Here's how the part is built. I have some questions about the finished solid (model axes, mm). A direction names the side the tool comes from. Round coordinates to 2 decimals unless told otherwise and drop trailing zeros. Write each loop counter-clockwise with the first axis right and the second up, starting at its lowest first coordinate (ties: lowest second). Pieces come first, ordered by that corner, then holes. Notation, with made-up numbers: (-17.75, 19) -> (5.25, 19) arc R25 ccw to (5.25, 51) -> close; hole circle Ø9 at (29.5, -4.75). An arc over 180 degrees is marked (long way). Answer in a Markdown table with one row per item. Add a question column.
from build123d import *

# Parameters (mm, degrees)
SKETCH_1_W          = 40
SKETCH_1_H          = 20
EXTRUDE_1_DEPTH     = 6
SKETCH_2_W          = 40
SKETCH_2_H          = 32.5
EXTRUDE_2_DEPTH     = 35
CUT_EXTRUDE_1_DEPTH = 13
CUT_EXTRUDE_2_DEPTH = 2
SKETCH_6_W          = 40
SKETCH_6_H          = 41
CUT_EXTRUDE_3_DEPTH = 5
SKETCH_8_R          = 1.7
CUT_EXTRUDE_4_DEPTH = 49.79805324
SKETCH_9_W          = 40
SKETCH_9_H          = 12.5
SKETCH_9_H_2        = 8
CUT_EXTRUDE_5_DEPTH = 41
CUT_EXTRUDE_6_DEPTH = 2
SKETCH_11_R         = 3.2
CUT_EXTRUDE_7_DEPTH = 2.8
SKETCH_12_W         = 0.4
SKETCH_12_H         = 41
CUT_EXTRUDE_8_DEPTH = 5


with BuildPart() as part:
    # Эскиз1 → Бобышка-Вытянуть1 (new body)
    with BuildSketch(Plane.XY):
        Rectangle(SKETCH_1_W, SKETCH_1_H)
    extrude(amount=EXTRUDE_1_DEPTH)

    # Эскиз2 → Бобышка-Вытянуть2 (add)
    with BuildSketch(Plane(origin=(0, 0, 0), x_dir=(-1, 0, 0), z_dir=(0, 0, -1))):
        with Locations((0, 6.25)):
            Rectangle(SKETCH_2_W, SKETCH_2_H)
    extrude(amount=EXTRUDE_2_DEPTH)

    # Эскиз3 → Вырез-Вытянуть1 (cut)
    with BuildSketch(Plane.XZ.offset(10)):
        Polygon((-7, 6), (-7, -1), (-9, -1), (-9, -23), (-6.5, -26), (-6.5, -33), (-4.5, -33), (-4.5, -35), (4.5, -35), (4.5, -33), (6.5, -33), (6.5, -26), (9, -23), (9, -1), (7, -1), (7, 6), align=None)
    extrude(amount=-CUT_EXTRUDE_1_DEPTH, mode=Mode.SUBTRACT)

    # Эскиз5 → Вырез-Вытянуть2 (cut)
    with BuildSketch(Plane.XZ.offset(-3)):
        Polygon((-9, -1), (9, -1), (9, -23), (6.5, -26), (6.5, -33), (-6.5, -33), (-6.5, -26), (-9, -23), align=None)
    extrude(amount=-CUT_EXTRUDE_2_DEPTH, mode=Mode.SUBTRACT)

    # Эскиз6 → Вырез-Вытянуть3 (cut)
    with BuildSketch(Plane.XZ.offset(10)):
        with Locations((0, -14.5)):
            Rectangle(SKETCH_6_W, SKETCH_6_H)
    extrude(amount=-CUT_EXTRUDE_3_DEPTH, mode=Mode.SUBTRACT)

    # Эскиз8 → Вырез-Вытянуть4 (cut, through all)
    with BuildSketch(Plane.XZ.offset(5)):
        with Locations((12, -26)):
            Circle(SKETCH_8_R)
        with Locations((14.5, -6)):
            Circle(SKETCH_8_R)
        with Locations(Location((-12, -26, 0), (0, 0, 180))):
            Circle(SKETCH_8_R)
        with Locations(Location((-14.5, -6, 0), (0, 0, 180))):
            Circle(SKETCH_8_R)
    extrude(amount=-CUT_EXTRUDE_4_DEPTH, mode=Mode.SUBTRACT)

    # Эскиз9 → Вырез-Вытянуть5 (cut)
    with BuildSketch(Plane.XY.offset(6)):
        with Locations((0, 16.25)):
            Rectangle(SKETCH_9_W, SKETCH_9_H)
        with Locations((0, -1)):
            Rectangle(SKETCH_9_W, SKETCH_9_H_2)
    extrude(amount=-CUT_EXTRUDE_5_DEPTH, mode=Mode.SUBTRACT)

    # Эскиз10 → Вырез-Вытянуть6 (cut)
    with BuildSketch(Plane.XZ.offset(-3)):
        Polygon((-20, 6), (-6.4, 6), (-6.4, -1), (-4, -33), (-4, -35), (-20, -35), align=None)
    cut_extrude_6 = extrude(amount=-CUT_EXTRUDE_6_DEPTH, mode=Mode.SUBTRACT)

    # Зеркальное отражение1: Вырез-Вытянуть6 across plane
    add(cut_extrude_6.mirror(Plane(origin=(0, 0, 0), x_dir=(0, 0, 1), z_dir=(1, 0, 0))), mode=Mode.SUBTRACT)

    # Эскиз11 → Вырез-Вытянуть7 (cut)
    with BuildSketch(Plane(origin=(0, 10, 0), x_dir=(1, 0, 0), z_dir=(0, 1, 0))):
        with Locations(Location((14.5, 6, 0), (0, 0, 180))):
            Circle(SKETCH_11_R)
        with Locations((-14.5, 6)):
            Circle(SKETCH_11_R)
        Polygon((-12, 29.233161507), (-14.8, 27.616580754), (-14.8, 24.383419246), (-12, 22.766838493), (-9.2, 24.383419246), (-9.2, 27.616580754), align=None)
        Polygon((9.2, 27.616580754), (12, 29.233161507), (14.8, 27.616580754), (14.8, 24.383419246), (12, 22.766838493), (9.2, 24.383419246), align=None)
    extrude(amount=-CUT_EXTRUDE_7_DEPTH, mode=Mode.SUBTRACT)

    # Эскиз12 → Вырез-Вытянуть8 (cut)
    with BuildSketch(Plane(origin=(0, 10, 0), x_dir=(1, 0, 0), z_dir=(0, 1, 0))):
        with Locations((-19.8, 14.5)):
            Rectangle(SKETCH_12_W, SKETCH_12_H)
        with Locations((19.8, 14.5)):
            Rectangle(SKETCH_12_W, SKETCH_12_H)
    extrude(amount=-CUT_EXTRUDE_8_DEPTH, mode=Mode.SUBTRACT)


solid = part.part
Item 1: I need wall thicknesses on line 1 along X through (y, z) = (6.25, -5.5); line 2 along Z through (x, y) = (12, 6.7); line 3 along Z through (x, y) = (-1.5, 3.75). Which ranges of each line are inside material? Lowest first, please. Write a range as from..to.
Item 2: If we section it at B-B on y = 8.75: Please give me the cut outline in (x, z).
Item 3: For P1, Ø1.6, axis at y = 4, z = -34.5, coming from the +X side; P2, Ø3, axis at x = -11, z = -25, coming from the -Y side; P3, Ø0.6, axis at y = 4, z = 1, coming from the -X side; P4, Ø4.5, axis at x = -11, z = -26, coming from the +Y side, each with a flat end and sliding along its axis, tell me the tip position at first contact or that it passes through.
Item 4: On a 3-axis mill with a long thin cutter (end or side, diameter ignored), from which of +Z, -Z, +X, -X, +Y, -Y can I reach the whole of each face in a straight line? I mean faces 4 (the flat face through (13.3, 7.2, -24.6)), 5 (the flat face through (0, 4, -33)), 6 (the cylindrical face through (12.914, 6.085, -24.567)). Say none if no direction works.
Item 5: If we section it at A-A on z = -26: Please give me the cut outline in (x, y), then the cut area to 3 significant figures.
Item 6: If we mould it in two halves opening along Z, with no side actions, what happens to faces 1 (the flat face through (6.4, 4, 3)), 2 (the flat face through (0, 4, -1)), 3 (the flat face through (0, 7, 6))? For each: pulls with the +Z half, pulls with the -Z half, needs draft (parallel to the pull), parting line crosses it, or undercut.
Item 7: If we section it at D-D on z = 1: Please give me the cut outline in (x, y), then the cut area to 3 significant figures.
Item 8: If we section it at C-C on x = 1: Please give me the cut outline in (y, z), then the cut area to 3 significant figures.
Results list:
| question | item | result |
|---|---|---|
| 1 | line 1 | -19.6..-16.12, -12.88..12.88, 16.12..19.6 |
| 1 | line 2 | -35..-27.7, -24.3..6 |
| 1 | line 3 | -35..-33, -1..6 |
| 2 | outline | (-19.6, -35) -> (19.6, -35) -> (19.6, 6) -> (-19.6, 6) -> close; hole circle Ø6.4 at (-14.5, -6); hole (-14.8, -27.62) -> (-12, -29.23) -> (-9.2, -27.62) -> (-9.2, -24.38) -> (-12, -22.77) -> (-14.8, -24.38) -> close; hole (9.2, -27.62) -> (12, -29.23) -> (14.8, -27.62) -> (14.8, -24.38) -> (12, -22.77) -> (9.2, -24.38) -> close; hole circle Ø6.4 at (14.5, -6) |
| 3 | P1 | x = 4 |
| 3 | P2 | y = 5 |
| 3 | P3 | x = -6.4 |
| 3 | P4 | y = 10 |
| 4 | face 4 | +Y |
| 4 | face 5 | +X, -X, -Y |
| 4 | face 6 | +Y, -Y |
| 5 | outline | (-19.6, 5) -> (-13.7, 5) -> (-13.7, 7.2) -> (-14.8, 7.2) -> (-14.8, 10) -> (-19.6, 10) -> close; (-10.3, 5) -> (10.3, 5) -> (10.3, 7.2) -> (9.2, 7.2) -> (9.2, 10) -> (-9.2, 10) -> (-9.2, 7.2) -> (-10.3, 7.2) -> close; (13.7, 5) -> (19.6, 5) -> (19.6, 10) -> (14.8, 10) -> (14.8, 7.2) -> (13.7, 7.2) -> close |
| 5 | area | 150 mm² |
| 6 | face 1 | needs draft |
| 6 | face 2 | undercut |
| 6 | face 3 | pulls with the +Z half |
| 7 | outline | (-19.6, 5) -> (-6.4, 5) -> (-6.4, 3) -> (6.4, 3) -> (6.4, 5) -> (19.6, 5) -> (19.6, 10) -> (-19.6, 10) -> close |
| 7 | area | 222 mm² |
| 8 | outline | (3, -35) -> (10, -35) -> (10, 6) -> (3, 6) -> (3, -1) -> (5, -1) -> (5, -33) -> (3, -33) -> close |
| 8 | area | 223 mm² |
